For this review, take the finished solid that the model builds, in its own axes (mm). Face numbers are marked on the shaded views. A direction names the side the tool comes from. Round coordinates to 2 decimals unless told otherwise and drop trailing zeros. Order: outer loops, then holes, each group sorted by start corner. A loop starts at its lowest first (then second) coordinate and runs counter-clockwise, first axis right, second up.
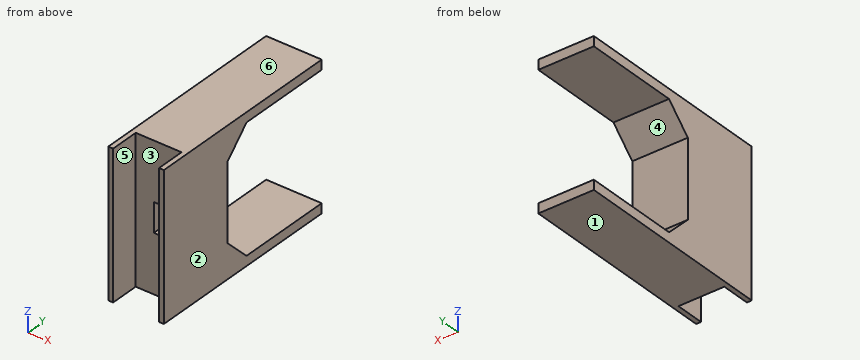
```python
from build123d import *

# Parameters (mm, degrees)
SKETCH1_W           = 11.5
SKETCH1_H           = 30
BOSS_EXTRUDE1_DEPTH = 11
SKETCH3_W           = 11.5
SKETCH3_H           = 30
BOSS_EXTRUDE3_DEPTH = 6
SKETCH4_W           = 9.5
SKETCH4_H           = 6
CUT_EXTRUDE1_DEPTH  = 33.466328711
SKETCH7_W           = 2
SKETCH7_H           = 6
CUT_EXTRUDE2_DEPTH  = 10
SKETCH8_W           = 11.5
SKETCH8_H           = 30
BOSS_EXTRUDE4_DEPTH = 25
SKETCH9_W           = 26
SKETCH9_H           = 25
CUT_EXTRUDE3_DEPTH  = 41.660177078
CHAMFER1_SIZE       = 5


with BuildPart() as part:
    # Sketch1 → Boss-Extrude1 (new body)
    with BuildSketch(Plane(origin=(0, 0, 0), x_dir=(1, 0, 0), z_dir=(0, 1, 0))):
        Rectangle(SKETCH1_W, SKETCH1_H)
    extrude(amount=BOSS_EXTRUDE1_DEPTH)

    # Sketch3 → Boss-Extrude3 (add)
    with BuildSketch(Plane.XZ):
        Rectangle(SKETCH3_W, SKETCH3_H)
    extrude(amount=BOSS_EXTRUDE3_DEPTH)

    # Sketch4 → Cut-Extrude1 (cut, through all)
    with BuildSketch(Plane.XY.offset(15)):
        with Locations((0, -3)):
            Rectangle(SKETCH4_W, SKETCH4_H)
    extrude(amount=-CUT_EXTRUDE1_DEPTH, mode=Mode.SUBTRACT)

    # Sketch7 → Cut-Extrude2 (cut)
    with BuildSketch(Plane.XZ):
        Rectangle(SKETCH7_W, SKETCH7_H)
    extrude(amount=-CUT_EXTRUDE2_DEPTH, mode=Mode.SUBTRACT)

    # Sketch8 → Boss-Extrude4 (add)
    with BuildSketch(Plane(origin=(0, 11, 0), x_dir=(1, 0, 0), z_dir=(0, 1, 0))):
        Rectangle(SKETCH8_W, SKETCH8_H)
    extrude(amount=BOSS_EXTRUDE4_DEPTH)

    # Sketch9 → Cut-Extrude3 (cut, through all)
    with BuildSketch(Plane.ZY.offset(5.75)):
        with Locations((0, 23.5)):
            Rectangle(SKETCH9_W, SKETCH9_H)
    extrude(amount=-CUT_EXTRUDE3_DEPTH, mode=Mode.SUBTRACT)

    # Chamfer1
    chamfer1_edges = [part.edges().sort_by_distance(p)[0] for p in [
        (0, 11, -13),
        (0, 11, 13),
    ]]
    chamfer(chamfer1_edges, length=CHAMFER1_SIZE)


solid = part.part
```
Q1. Mouldability with a two-part tool opening along X and no side actions: class the marked faces 1, 2 and 3 as +X half, -X half, draft (parallel to the pull), parting line (faces both ways), or undercut.
Q2. Tool access review of the marked faces 4, 5 and 6: name each direction out of +Z, -Z, +X, -X, +Y, -Y from which nothing blocks a thin tool from reaching the whole face with its end or side.
Q3. Take a section at A-A, the plane y = -0.5. State the section outline as (x, z) points, plus the area to 3 significant figures.
Q4. Take a section at B-B, the plane x = -0.25. State the section outline as (y, z) points, plus the area to 3 significant figures.
Q5. Take a section at C-C, the plane y = 13.5. State the section outline as (x, z) points, plus the area to 4 significant figures.
Q6. Clearance check with flat-ended pins moving along their axes: pin 1 (0.6 mm diameter, centred on x = 0.5, z = -1.5, fed in from -Y); pin 2 (3.5 mm diameter, centred on x = 2.5, z = -0.5, fed in from +Y); pin 3 (6 mm diameter, centred on x = -3.5, z = -5.5, fed in from +Y). State where each tip first meets the part, or that it passes through.
Q7. Take a section at D-D, the plane z = -0.5. State the section outline as (x, y) points, plus the area to 4 significant figures.
Q8. Wall thickness on line 1 (X direction, y = -4, z = 6.25); line 2 (Y direction, x = -1.75, z = -5); line 3 (Y direction, x = -4, z = -10): over which ranges is each line inside the solid? List them lowest first.
Working result:
1. face 1: draft
1. face 2: +X half
1. face 3: undercut
2. face 4: +X, -X, +Y
2. face 5: +Z, -Z, -Y
2. face 6: +Z, +X, -X, +Y, -Y
3. outline: (-5.75, -15) - (-4.75, -15) - (-4.75, 15) - (-5.75, 15) - close; (4.75, -15) - (5.75, -15) - (5.75, 15) - (4.75, 15) - close
3. area: 60.0 mm2
4. outline: (0, -15) - (36, -15) - (36, -13) - (16, -13) - (11, -8) - (11, 8) - (16, 13) - (36, 13) - (36, 15) - (0, 15) - (0, 3) - (10, 3) - (10, -3) - (0, -3) - close
4. area: 395 mm2
5. outline: (-5.75, -15) - (5.75, -15) - (5.75, -10.5) - (-5.75, -10.5) - close; (-5.75, 10.5) - (5.75, 10.5) - (5.75, 15) - (-5.75, 15) - close
5. area: 103.5 mm2
6. pin 1: stops at y = 10
6. pin 2: stops at y = 11
6. pin 3: stops at y = 11.5
7. outline: (-5.75, -6) - (-4.75, -6) - (-4.75, 0) - (-1, 0) - (-1, 10) - (1, 10) - (1, 0) - (4.75, 0) - (4.75, -6) - (5.75, -6) - (5.75, 11) - (-5.75, 11) - close
7. area: 118.5 mm2
8. line 1: x = -5.75 to -4.75, 4.75 to 5.75
8. line 2: y = 0 to 11
8. line 3: y = 0 to 13
